For this review, use the dimensioned drawing (mm, ordinates from the lowest corner) and the shaded views. A direction names the side the tool comes from. Coordinates: 2 decimals unless noted, no trailing zeros. Loops run counter-clockwise (first coordinate to the right, second up) from the corner with the lowest first, then second, coordinate; pieces in that order, holes last.
1. Clearance check with flat-ended pins moving along their axes: P1, Ø1.5, axis at x = 2.5, z = 3, coming from the +Y side; P2, Ø2, axis at y = 0.5, z = 3.5, coming from the -X side; P3, Ø1.5, axis at y = 2.5, z = 1.5, coming from the +X side. State where each tip first meets the part, or that it passes through.
2. Take a section at B-B, the plane x = 2.75. State the section outline as (y, z) points, then the cut area to 4 significant figures.
3. Take a section at D-D, the plane y = 1.55. State the section outline as (x, z) points, then the cut area to 3 significant figures.
4. Machinability: for the marked faces 1, 2 and 3, which of the approach directions +Z, -Z, +X, -X, +Y, -Y give a long, thin tool a straight path to every point of the face, cutting with its end or side? Answer none if there is none.
5. Take a section at A-A, the plane y = 2.9. State the section outline as (x, z) points.
6. Take a section at C-C, the plane z = 2.2. State the section outline as (x, y) points.
7. To check wall thickness, follow probe 1 along X at (y, z) = (1.55, 1.45); probe 2 along Y at (x, z) = (2.7, 3.1). State the ranges of each line that lie inside material, in increasing order.
8. Mouldability with a two-part tool opening along X and no side actions: class the marked faces 4, 5 and 6 as pulls with the +X half, pulls with the -X half, needs draft (parallel to the pull), parting line crosses it, or undercut.
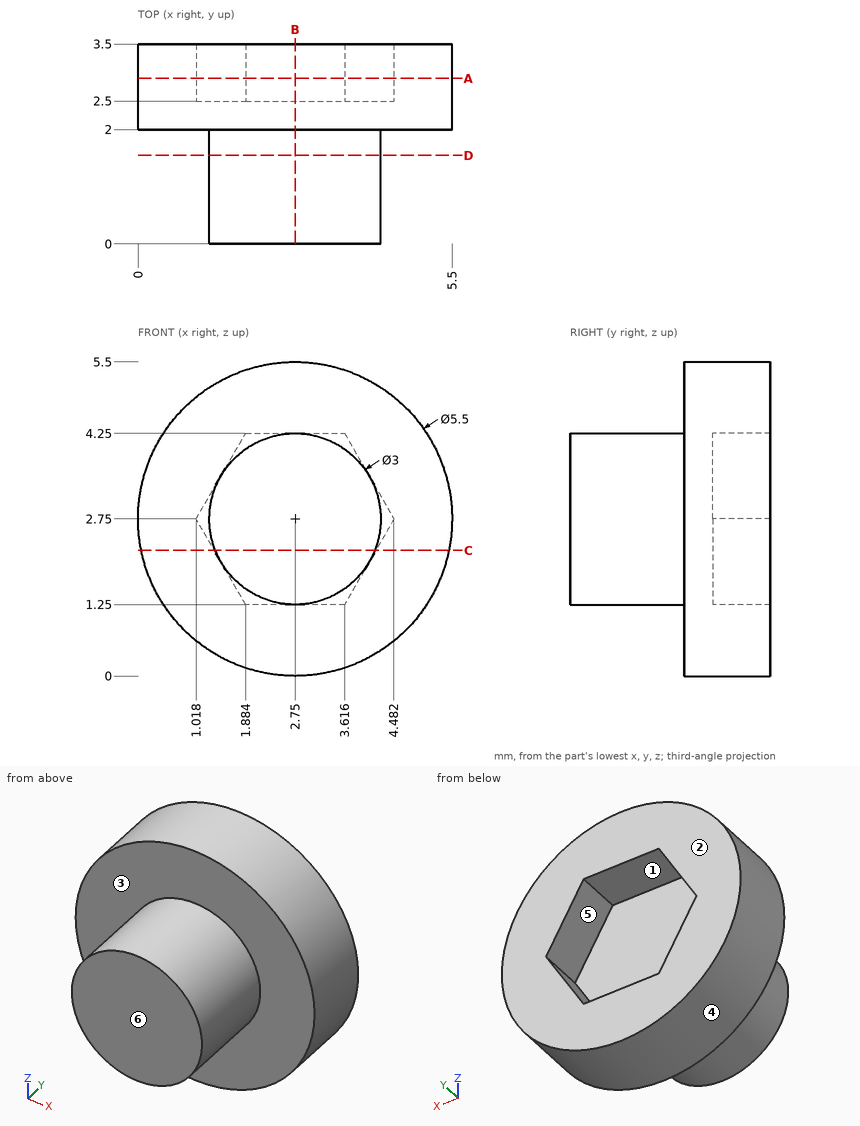
Results list:
1. P1: stops at y = 2.5
1. P2: stops at x = 1.25
1. P3: stops at x = 5.45
2. outline: (0, 1.25) - (2, 1.25) - (2, 0) - (3.5, 0) - (3.5, 1.25) - (2.5, 1.25) - (2.5, 4.25) - (3.5, 4.25) - (3.5, 5.5) - (2, 5.5) - (2, 4.25) - (0, 4.25) - close
2. area: 11.25 mm2
3. outline: circle Ø3 at (2.75, 2.75)
3. area: 7.07 mm2
4. face 1: +Y
4. face 2: +Z, -Z, +X, -X, +Y
4. face 3: -Y
5. outline: circle Ø5.5 at (2.75, 2.75); hole (1.02, 2.75) - (1.88, 1.25) - (3.62, 1.25) - (4.48, 2.75) - (3.62, 4.25) - (1.88, 4.25) - close
6. outline: (0.06, 2) - (1.35, 2) - (1.35, 0) - (4.15, 0) - (4.15, 2) - (5.44, 2) - (5.44, 3.5) - (4.16, 3.5) - (4.16, 2.5) - (1.34, 2.5) - (1.34, 3.5) - (0.06, 3.5) - close
7. probe 1: x = 2 to 3.5
7. probe 2: y = 0 to 2.5
8. face 4: parting line crosses it
8. face 5: undercut
8. face 6: needs draft
